Work out the finished part from the listing and answer in its coordinate system (mm). Face numbers are marked on the shaded views. A direction names the side the tool comes from. Give positions to 0.01 mm unless a question says otherwise; leave off trailing zeros. Order: outer loops, then holes, each group sorted by start corner. A loop starts at its lowest first (then second) coordinate and runs counter-clockwise, first axis right, second up. Notation, with made-up numbers: (-35.75, 9) - (-9.75, 9) arc R23 ccw to (-9.75, 43) - close; hole circle Ø11 at (-19.5, 59). An arc over 180 degrees is marked (long way). Put each result on its own line as item: value.
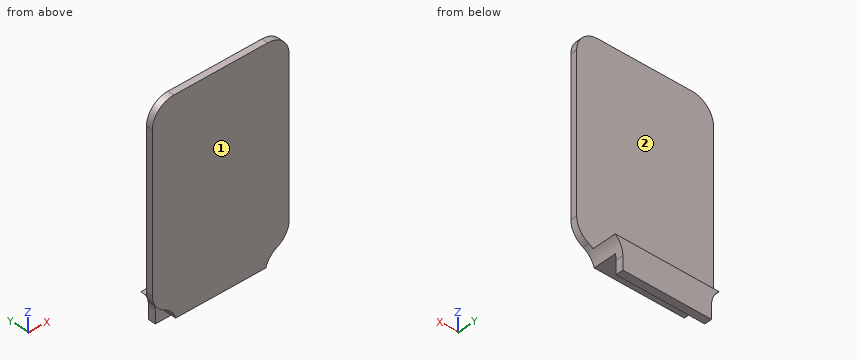
```python
from build123d import *

# Parameters (mm, degrees)
SKETCH1_W           = 41.5
SKETCH1_H           = 92.8
BOSS_EXTRUDE1_DEPTH = 3
SKETCH2_W           = 5
SKETCH2_H           = 3.5
SKETCH2_H_2         = 7.9
SKETCH2_W_2         = 9
BOSS_EXTRUDE2_DEPTH = 41.5
SKETCH3_W           = 64.02
SKETCH3_H           = 92.8
BOSS_EXTRUDE3_DEPTH = 3
FILLET1_R           = 10
FILLET2_R           = 10


with BuildPart() as part:
    # Sketch1 → Boss-Extrude1 (new body)
    with BuildSketch(Plane(origin=(0, 0, 0), x_dir=(1, 0, 0), z_dir=(0, 1, 0))):
        with Locations((32.680302971, 6.528754522)):
            Rectangle(SKETCH1_W, SKETCH1_H)
    extrude(amount=BOSS_EXTRUDE1_DEPTH)

    # Sketch2 → Boss-Extrude2 (add)
    with BuildSketch(Plane(origin=(53.430302971, 0, 0), x_dir=(0, 0, -1), z_dir=(1, 0, 0))):
        with Locations((50.428754522, 12.65)):
            Rectangle(SKETCH2_W, SKETCH2_H)
        with Locations((50.428754522, 6.95)):
            Rectangle(SKETCH2_W, SKETCH2_H_2)
        with Locations((57.428754522, 12.65)):
            Rectangle(SKETCH2_W_2, SKETCH2_H)
    extrude(amount=-BOSS_EXTRUDE2_DEPTH)

    # Sketch3 → Boss-Extrude3 (add)
    with BuildSketch(Plane(origin=(0, 3, 0), x_dir=(1, 0, 0), z_dir=(0, 1, 0))):
        with Locations((32.680302971, 1.195086087)):
            Rectangle(SKETCH3_W, SKETCH3_H)
    extrude(amount=-BOSS_EXTRUDE3_DEPTH)

    # Fillet1
    fillet1_edges = [part.edges().sort_by_distance(p)[0] for p in [
        (0.670302971, 1.5, -47.595086087),
        (64.690302971, 1.5, -47.595086087),
        (64.690302971, 1.5, 45.204913913),
        (0.670302971, 1.5, 45.204913913),
    ]]
    fillet(fillet1_edges, radius=FILLET1_R)

    # Fillet2
    # the kernel refuses this fillet: 10 mm, written as the material it adds along each edge
    with BuildSketch(Plane(origin=(11.930302971, 22.973075278, -47.595086087), x_dir=(0, 0, -1), z_dir=(0, -1, 0))) as fillet2_piece_1_section:
        with BuildLine():
            CenterArc((7.989230111, -10), FILLET2_R, 90, 64.087374577)
            Line((-1.005384944, -5.63), (-1.90484645, -5.193))
            ThreePointArc((-1.90484645, -5.193), (-1, -1.26), (-1, 0))
            Line((-1, 0), (0, 1))
            Line((0, 1), (7.989230111, 1))
            Line((7.989230111, 1), (7.989230111, 0))
        make_face()
    fillet2_piece_1 = extrude(amount=22.973075278, mode=Mode.PRIVATE)
    fillet2_piece_1 = split(fillet2_piece_1, bisect_by=Plane(origin=(12.365804392, 12.65, -52.928754522), z_dir=(0, 0, -1)), keep=Keep.TOP, mode=Mode.PRIVATE)
    fillet2_piece_1 = split(fillet2_piece_1, bisect_by=Plane(origin=(12.365804392, 10.9, -54.185779558), z_dir=(0, 1, 0)), keep=Keep.TOP, mode=Mode.PRIVATE)
    fillet2_piece_1 = split(fillet2_piece_1, bisect_by=Plane(origin=(12.365804392, 14.4, -54.185779558), z_dir=(0, -1, 0)), keep=Keep.TOP, mode=Mode.PRIVATE)
    add(fillet2_piece_1)
    with BuildSketch(Plane(origin=(11.930302971, 22.973075278, -47.595086087), x_dir=(0, 0, -1), z_dir=(0, -1, 0))) as fillet2_piece_2_section:
        with BuildLine():
            CenterArc((7.989230111, -10), FILLET2_R, 90, 64.087374577)
            Line((-1.005384944, -5.63), (-1.90484645, -5.193))
            ThreePointArc((-1.90484645, -5.193), (-1, -1.26), (-1, 0))
            Line((-1, 0), (0, 1))
            Line((0, 1), (7.989230111, 1))
            Line((7.989230111, 1), (7.989230111, 0))
        make_face()
    fillet2_piece_2 = extrude(amount=22.973075278, mode=Mode.PRIVATE)
    fillet2_piece_2 = split(fillet2_piece_2, bisect_by=Plane(origin=(11.467639637, 12.65, -52.928754522), z_dir=(0, 0, 1)), keep=Keep.TOP, mode=Mode.PRIVATE)
    fillet2_piece_2 = split(fillet2_piece_2, bisect_by=Plane(origin=(11.467639637, 10.9, -49.92895082), z_dir=(0, 1, 0)), keep=Keep.TOP, mode=Mode.PRIVATE)
    fillet2_piece_2 = split(fillet2_piece_2, bisect_by=Plane(origin=(11.467639637, 14.4, -49.92895082), z_dir=(0, -1, 0)), keep=Keep.TOP, mode=Mode.PRIVATE)
    fillet2_piece_2 = split(fillet2_piece_2, bisect_by=Plane(origin=(11.467639637, 12.65, -47.928754522), z_dir=(0, 0, -1)), keep=Keep.TOP, mode=Mode.PRIVATE)
    add(fillet2_piece_2)
    with BuildSketch(Plane(origin=(11.930302971, 22.973075278, -47.595086087), x_dir=(0, 0, -1), z_dir=(0, -1, 0))) as fillet2_piece_3_section:
        with BuildLine():
            CenterArc((7.989230111, -10), FILLET2_R, 90, 64.087374577)
            Line((-1.005384944, -5.63), (-1.90484645, -5.193))
            ThreePointArc((-1.90484645, -5.193), (-1, -1.26), (-1, 0))
            Line((-1, 0), (0, 1))
            Line((0, 1), (7.989230111, 1))
            Line((7.989230111, 1), (7.989230111, 0))
        make_face()
    fillet2_piece_3 = extrude(amount=22.973075278, mode=Mode.PRIVATE)
    fillet2_piece_3 = split(fillet2_piece_3, bisect_by=Plane(origin=(11.467639637, 6.95, -52.928754522), z_dir=(0, 0, 1)), keep=Keep.TOP, mode=Mode.PRIVATE)
    fillet2_piece_3 = split(fillet2_piece_3, bisect_by=Plane(origin=(11.467639637, 10.9, -49.92895082), z_dir=(0, -1, 0)), keep=Keep.TOP, mode=Mode.PRIVATE)
    fillet2_piece_3 = split(fillet2_piece_3, bisect_by=Plane(origin=(11.467639637, 6.95, -47.928754522), z_dir=(0, 0, -1)), keep=Keep.TOP, mode=Mode.PRIVATE)
    fillet2_piece_3 = split(fillet2_piece_3, bisect_by=Plane(origin=(11.467639637, 3, -49.92895082), z_dir=(0, 1, 0)), keep=Keep.TOP, mode=Mode.PRIVATE)
    add(fillet2_piece_3)
    with BuildSketch(Plane(origin=(11.930302971, 3, -47.595086087), x_dir=(0, 0, -1), z_dir=(0, -1, 0))) as fillet2_piece_4_section:
        with BuildLine():
            CenterArc((7.989230111, -10), FILLET2_R, 90, 64.087374577)
            Line((-1.005384944, -5.63), (-1.90484645, -5.193))
            ThreePointArc((-1.90484645, -5.193), (-1, -1.26), (-1, 0))
            Line((-1, 0), (0, 1))
            Line((0, 1), (7.989230111, 1))
            Line((7.989230111, 1), (7.989230111, 0))
        make_face()
    fillet2_piece_4 = extrude(amount=3, mode=Mode.PRIVATE)
    fillet2_piece_4 = split(fillet2_piece_4, bisect_by=Plane(origin=(11.467639637, 1.5, -52.928754522), z_dir=(0, 0, 1)), keep=Keep.TOP, mode=Mode.PRIVATE)
    fillet2_piece_4 = split(fillet2_piece_4, bisect_by=Plane(origin=(11.467639637, 1.5, -47.928754522), z_dir=(0, 0, -1)), keep=Keep.TOP, mode=Mode.PRIVATE)
    add(fillet2_piece_4)
    with BuildSketch(Plane(origin=(11.930302971, 3, -47.595086087), x_dir=(0, 0, -1), z_dir=(0, -1, 0))) as fillet2_piece_5_section:
        with BuildLine():
            CenterArc((7.989230111, -10), FILLET2_R, 90, 64.087374577)
            Line((-1.005384944, -5.63), (-1.90484645, -5.193))
            ThreePointArc((-1.90484645, -5.193), (-1, -1.26), (-1, 0))
            Line((-1, 0), (0, 1))
            Line((0, 1), (7.989230111, 1))
            Line((7.989230111, 1), (7.989230111, 0))
        make_face()
    fillet2_piece_5 = extrude(amount=3, mode=Mode.PRIVATE)
    fillet2_piece_5 = split(fillet2_piece_5, bisect_by=Plane(origin=(9.548517713, 1.5, -47.928754522), z_dir=(0, 0, 1)), keep=Keep.TOP, mode=Mode.PRIVATE)
    add(fillet2_piece_5)
    with BuildSketch(Plane(origin=(53.430302971, 0, -47.595086087), x_dir=(0.9844267342530738, 0, 0.17579534944880632), z_dir=(0, 1, 0))) as fillet2_piece_6_section:
        with BuildLine():
            CenterArc((8.439797843, 9.622765202), FILLET2_R, 190.124945844, 64.087374577)
            Line((-1.404469499, 7.864811708), (-2.388896234, 7.689016358))
            Line((-2.388896234, 7.689016358), (-0.984426734, -0.175795349))
            Line((-0.984426734, -0.175795349), (0.175795349, -0.984426734))
            ThreePointArc((0.175795349, -0.984426734), (1.416173035, -0.762924594), (5.446991178, -0.96227652))
            Line((5.446991178, -0.96227652), (5.719064511, 0))
        make_face()
    fillet2_piece_6 = extrude(amount=3, mode=Mode.PRIVATE)
    fillet2_piece_6 = split(fillet2_piece_6, bisect_by=Plane(origin=(55.812088229, 1.5, -47.928754522), z_dir=(0, 0, 1)), keep=Keep.TOP, mode=Mode.PRIVATE)
    add(fillet2_piece_6)
    with BuildSketch(Plane(origin=(53.430302971, 0, -47.595086087), x_dir=(0.9844267342530738, 0, 0.17579534944880632), z_dir=(0, 1, 0))) as fillet2_piece_7_section:
        with BuildLine():
            CenterArc((8.439797843, 9.622765202), FILLET2_R, 190.124945844, 64.087374577)
            Line((-1.404469499, 7.864811708), (-2.388896234, 7.689016358))
            Line((-2.388896234, 7.689016358), (-0.984426734, -0.175795349))
            Line((-0.984426734, -0.175795349), (0.175795349, -0.984426734))
            ThreePointArc((0.175795349, -0.984426734), (1.416173035, -0.762924594), (5.446991178, -0.96227652))
            Line((5.446991178, -0.96227652), (5.719064511, 0))
        make_face()
    fillet2_piece_7 = extrude(amount=3, mode=Mode.PRIVATE)
    fillet2_piece_7 = split(fillet2_piece_7, bisect_by=Plane(origin=(53.892966305, 1.5, -52.928754522), z_dir=(0, 0, 1)), keep=Keep.TOP, mode=Mode.PRIVATE)
    fillet2_piece_7 = split(fillet2_piece_7, bisect_by=Plane(origin=(53.892966305, 1.5, -47.928754522), z_dir=(0, 0, -1)), keep=Keep.TOP, mode=Mode.PRIVATE)
    add(fillet2_piece_7)
    with BuildSketch(Plane(origin=(53.430302971, 0, -47.595086087), x_dir=(0.9844267342530738, 0, 0.17579534944880632), z_dir=(0, 1, 0))) as fillet2_piece_8_section:
        with BuildLine():
            CenterArc((8.439797843, 9.622765202), FILLET2_R, 190.124945844, 64.087374577)
            Line((-1.404469499, 7.864811708), (-2.388896234, 7.689016358))
            Line((-2.388896234, 7.689016358), (-0.984426734, -0.175795349))
            Line((-0.984426734, -0.175795349), (0.175795349, -0.984426734))
            ThreePointArc((0.175795349, -0.984426734), (1.416173035, -0.762924594), (5.446991178, -0.96227652))
            Line((5.446991178, -0.96227652), (5.719064511, 0))
        make_face()
    fillet2_piece_8 = extrude(amount=22.973075278, mode=Mode.PRIVATE)
    fillet2_piece_8 = split(fillet2_piece_8, bisect_by=Plane(origin=(53.892966305, 3, -49.92895082), z_dir=(0, 1, 0)), keep=Keep.TOP, mode=Mode.PRIVATE)
    fillet2_piece_8 = split(fillet2_piece_8, bisect_by=Plane(origin=(53.892966305, 6.95, -52.928754522), z_dir=(0, 0, 1)), keep=Keep.TOP, mode=Mode.PRIVATE)
    fillet2_piece_8 = split(fillet2_piece_8, bisect_by=Plane(origin=(53.892966305, 6.95, -47.928754522), z_dir=(0, 0, -1)), keep=Keep.TOP, mode=Mode.PRIVATE)
    fillet2_piece_8 = split(fillet2_piece_8, bisect_by=Plane(origin=(53.892966305, 10.9, -49.92895082), z_dir=(0, -1, 0)), keep=Keep.TOP, mode=Mode.PRIVATE)
    add(fillet2_piece_8)
    with BuildSketch(Plane(origin=(53.430302971, 0, -47.595086087), x_dir=(0.9844267342530738, 0, 0.17579534944880632), z_dir=(0, 1, 0))) as fillet2_piece_9_section:
        with BuildLine():
            CenterArc((8.439797843, 9.622765202), FILLET2_R, 190.124945844, 64.087374577)
            Line((-1.404469499, 7.864811708), (-2.388896234, 7.689016358))
            Line((-2.388896234, 7.689016358), (-0.984426734, -0.175795349))
            Line((-0.984426734, -0.175795349), (0.175795349, -0.984426734))
            ThreePointArc((0.175795349, -0.984426734), (1.416173035, -0.762924594), (5.446991178, -0.96227652))
            Line((5.446991178, -0.96227652), (5.719064511, 0))
        make_face()
    fillet2_piece_9 = extrude(amount=22.973075278, mode=Mode.PRIVATE)
    fillet2_piece_9 = split(fillet2_piece_9, bisect_by=Plane(origin=(53.892966305, 12.65, -52.928754522), z_dir=(0, 0, 1)), keep=Keep.TOP, mode=Mode.PRIVATE)
    fillet2_piece_9 = split(fillet2_piece_9, bisect_by=Plane(origin=(53.892966305, 12.65, -47.928754522), z_dir=(0, 0, -1)), keep=Keep.TOP, mode=Mode.PRIVATE)
    fillet2_piece_9 = split(fillet2_piece_9, bisect_by=Plane(origin=(53.892966305, 14.4, -49.92895082), z_dir=(0, -1, 0)), keep=Keep.TOP, mode=Mode.PRIVATE)
    fillet2_piece_9 = split(fillet2_piece_9, bisect_by=Plane(origin=(53.892966305, 10.9, -49.92895082), z_dir=(0, 1, 0)), keep=Keep.TOP, mode=Mode.PRIVATE)
    add(fillet2_piece_9)
    with BuildSketch(Plane(origin=(53.430302971, 0, -47.595086087), x_dir=(0.9844267342530738, 0, 0.17579534944880632), z_dir=(0, 1, 0))) as fillet2_piece_10_section:
        with BuildLine():
            CenterArc((8.439797843, 9.622765202), FILLET2_R, 190.124945844, 64.087374577)
            Line((-1.404469499, 7.864811708), (-2.388896234, 7.689016358))
            Line((-2.388896234, 7.689016358), (-0.984426734, -0.175795349))
            Line((-0.984426734, -0.175795349), (0.175795349, -0.984426734))
            ThreePointArc((0.175795349, -0.984426734), (1.416173035, -0.762924594), (5.446991178, -0.96227652))
            Line((5.446991178, -0.96227652), (5.719064511, 0))
        make_face()
    fillet2_piece_10 = extrude(amount=22.973075278, mode=Mode.PRIVATE)
    fillet2_piece_10 = split(fillet2_piece_10, bisect_by=Plane(origin=(52.99480155, 12.65, -52.928754522), z_dir=(0, 0, -1)), keep=Keep.TOP, mode=Mode.PRIVATE)
    fillet2_piece_10 = split(fillet2_piece_10, bisect_by=Plane(origin=(52.99480155, 14.4, -54.185779558), z_dir=(0, -1, 0)), keep=Keep.TOP, mode=Mode.PRIVATE)
    fillet2_piece_10 = split(fillet2_piece_10, bisect_by=Plane(origin=(52.99480155, 10.9, -54.185779558), z_dir=(0, 1, 0)), keep=Keep.TOP, mode=Mode.PRIVATE)
    add(fillet2_piece_10)


solid = part.part
```
(1) Section C-C, the plane z = -25.5 is taken. Write down the section's boundary in (x, y).
Geometry check:
outline: (0.67, 0) - (64.69, 0) - (64.69, 3) - (0.67, 3) - close
(2) Section A-A, the plane y = 12 is taken. Write down the section's boundary in (x, z).
Geometry check:
outline: (8.36, -47.93) arc R10 cw to (11.93, -55.58) - (11.93, -61.93) - (53.43, -61.93) - (53.43, -55.58) arc R10 cw to (57, -47.93) - close
(3) Given pin 1 (6 mm diameter, centred on x = 43, y = 12, fed in from +Z); pin 2 (5.5 mm diameter, centred on x = 42.5, y = 8, fed in from -Z); pin 3 (3 mm diameter, centred on x = 8.5, z = -3.5, fed in from +Y), each flat-ended and moving along its own axis, determine where each tip first touches the part or whether it passes through.
Geometry check:
pin 1: stops at z = -47.93
pin 2: stops at z = -52.93
pin 3: stops at y = 3
(4) Section B-B, the plane x = 33 is taken. Write down the section's boundary in (y, z).
Geometry check:
outline: (0, -52.93) - (10.9, -52.93) - (10.9, -61.93) - (14.4, -61.93) - (14.4, -47.93) - (3, -47.93) - (3, 45.2) - (0, 45.2) - close
(5) Section D-D, the plane y = 1.5 is taken. Write down the section's boundary in (x, z), then the cut area to 3 significant figures.
Geometry check:
outline: (0.67, -37.6) arc R10 ccw to (6.3, -46.59) arc R10 cw to (11.57, -52.93) - (53.79, -52.93) arc R10 cw to (59.06, -46.59) arc R10 ccw to (64.69, -37.6) - (64.69, 35.2) arc R10 ccw to (54.69, 45.2) - (10.67, 45.2) arc R10 ccw to (0.67, 35.2) - close
area: 6,100 mm²
(6) A tool of negligible diameter and unlimited length cuts with its end or side. For the marked faces 1 and 2, from which of +Z, -Z, +X, -X, +Y, -Y can it reach the whole face along a straight path? Write none if from no direction.
Geometry check:
face 1: +Z, -Z, +X, -X, -Y
face 2: +Z, +X, -X, +Y
(7) Straight lines are drawn through the part: line 1 (Y direction, x = 4, z = 37.5); line 2 (Z direction, x = 22, y = 4.5); line 3 (Z direction, x = 38, y = 1.5). For each, find the intervals that lie inside material, in ascending order.
Geometry check:
line 1: y = 0 to 3
line 2: z = -52.93 to -47.93
line 3: z = -52.93 to 45.2
